```python
from build123d import *

# Parameters (mm, degrees)
CUT_EXTRUDE2_DEPTH      = 111.624951977
CUT_EXTRUDE2_DEPTH_BACK = 111.624951977
SKETCH2_W               = 40
SKETCH2_H               = 20
CUT_EXTRUDE3_DEPTH      = 110.603284622
CUT_EXTRUDE3_DEPTH_BACK = 110.603284622
SKETCH3_R               = 15


with BuildPart() as part:
    # Sketch1 → Revolve1 (revolve)
    with BuildSketch(Plane.XY):
        Polygon((0, 0), (-76.2, 0), (-76.2, 25), (-71.2, 25), (-71.2, 5), (0, 5), align=None)
    revolve(axis=Axis((0, 5, 0), (0, -1, 0)))

    # Sketch2 → Cut-Extrude2 (cut, two sides: drawn at the far end of the back side and taken through both)
    with BuildSketch(Plane(origin=(0, 0, 0), x_dir=(0, 0, -1), z_dir=(1, 0, 0)).offset(-CUT_EXTRUDE2_DEPTH_BACK)):
        with Locations((0, 15)):
            Rectangle(SKETCH2_W, SKETCH2_H)
    extrude(amount=CUT_EXTRUDE2_DEPTH + CUT_EXTRUDE2_DEPTH_BACK, mode=Mode.SUBTRACT)

    # Sketch3 → Cut-Extrude3 (cut, two sides: drawn at the far end of the back side and taken through both)
    with BuildSketch(Plane(origin=(0, 5, 0), x_dir=(1, 0, 0), z_dir=(0, 1, 0)).offset(-CUT_EXTRUDE3_DEPTH_BACK)):
        with Locations(Location((0, 0, 0), (0, 0, 180))):
            Circle(SKETCH3_R)
    extrude(amount=CUT_EXTRUDE3_DEPTH + CUT_EXTRUDE3_DEPTH_BACK, mode=Mode.SUBTRACT)


solid = part.part
```
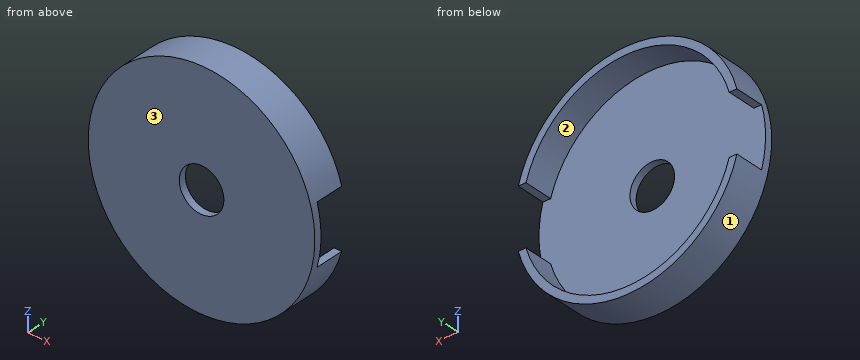
For this review, take the finished solid that the model builds, in its own axes (mm). Face numbers are marked on the shaded views. Coordinates: 2 decimals unless noted, no trailing zeros. Write each loop counter-clockwise with the first axis right and the second up, starting at its lowest first coordinate (ties: lowest second). Pieces come first, ordered by that corner, then holes. Notation, with made-up numbers: (32, -37) - (36, -37) arc R18 cw to (36, -20) - close; hole circle Ø11 at (44, 42.25). An arc over 180 degrees is marked (long way). Put each result on its own line as item: value.
1. For pin 1 (6 mm diameter, centred on x = 30, z = -33.5, fed in from +Y); pin 2 (3 mm diameter, centred on x = 0.5, y = 21, fed in from -Z); pin 3 (4 mm diameter, centred on x = 72, y = 11.5, fed in from +Z); pin 4 (2 mm diameter, centred on x = -47.5, y = 16, fed in from +Z), all flat-tipped, find the tip position at first contact; note any pin that passes through.
Values found:
pin 1: y = 5
pin 2: z = -76.2
pin 3: z = 30.11
pin 4: z = 60.37
2. Add section C-C, the plane y = 2. Give the boundary of the cut face in (x, z), then the cut area to 3 significant figures.
Values found:
outline: circle Ø152.4 at (0, 0); hole circle Ø30 at (0, 0)
area: 17,500 mm²
3. Add section B-B, the plane x = 0. Give the boundary of the cut face in (y, z), then the cut area to 3 significant figures.
Values found:
outline: (0, -76.2) - (25, -76.2) - (25, -71.2) - (5, -71.2) - (5, -15) - (0, -15) - close; (0, 15) - (5, 15) - (5, 71.2) - (25, 71.2) - (25, 76.2) - (0, 76.2) - close
area: 812 mm²
4. Wall thickness on probe 1 along Z at (x, y) = (0, 3.1); probe 2 along Y at (x, z) = (-7, 26.5): over which ranges is each line inside the solid? List them lowest first.
Values found:
probe 1: -76.2 to -15, 15 to 76.2
probe 2: 0 to 5
5. Add section D-D, the plane x = -61.5. Give the boundary of the cut face in (y, z).
Values found:
outline: (0, -44.99) - (25, -44.99) - (25, -35.88) - (5, -35.88) - (5, 35.88) - (25, 35.88) - (25, 44.99) - (0, 44.99) - close
6. Mouldability with a two-part tool opening along X and no side actions: class the marked faces 1, 2 and 3 as released by +X, released by -X, zero draft, split by the parting line, or undercut.
Values found:
face 1: split by the parting line
face 2: undercut
face 3: zero draft
7. Add section A-A, the plane z = 0. Give the boundary of the cut face in (x, y).
Values found:
outline: (-76.2, 0) - (-15, 0) - (-15, 5) - (-76.2, 5) - close; (15, 0) - (76.2, 0) - (76.2, 5) - (15, 5) - close
